Solid Edge part; units mm, degrees
sketch "Sketch1" plane through (0, 0, 0) normal (0, -1, 0) x (1, 0, 0)
  line L0 (38.9305, 51.9251) -> (68.9305, 51.9251)
  line L1 (68.9305, 51.9251) -> (68.9305, 21.9251)
  line L2 (68.9305, 21.9251) -> (38.9305, 21.9251)
  line L3 (38.9305, 21.9251) -> (38.9305, 51.9251)
  dimension "D1" = 38.9305
  dimension "D2" = 68.9305
extrude "Protrusion1" add sketch "Sketch1" against normal blind 15
sketch "Sketch2" plane through (63.9305, 0, 41.9251) normal (0, -1, 0) x (1, 0, 0)
  line L0 (-8, -5) -> (-8, -10)
  arc A0 (-8, -10) -> (-12, -10) centre (-10, -10) cw
  line L1 (-12, -10) -> (-12, -5)
  arc A1 (-12, -5) -> (-17, 0) centre (-17, -5) ccw
  line L2 (-17, 0) -> (-22, 0)
  arc A2 (-22, 0) -> (-22, 4) centre (-22, 2) cw
  line L3 (-22, 4) -> (-17, 4)
  arc A3 (-17, 4) -> (-14, 7) centre (-17, 7) ccw
  arc A4 (-14, 7) -> (-6, 7) centre (-10, 2.4867) cw
  arc A5 (-3, 4) -> (-6, 7) centre (-3, 7) cw
  line L4 (2, 4) -> (-3, 4)
  arc A6 (2, 0) -> (2, 4) centre (2, 2) ccw
  line L5 (-3, 0) -> (2, 0)
  arc A7 (-8, -5) -> (-3, 0) centre (-3, -5) cw
  dimension "D1" = 8
  dimension "D2" = 12
  dimension "D3" = 3
  dimension "D4" = 17
  dimension "D5" = 22
  dimension "D6" = 2
extrude "ExtrudedCutout_4" cut sketch "Sketch2" against normal blind 5
sketch "Sketch3" plane through (63.9305, 5, 35.4251) normal (0, -1, 0) x (1, 0, 0)
  circle A0 centre (-10, 8.5) radius 2.5
extrude "ExtrudedProtrusion_3" add sketch "Sketch3" along normal blind 5
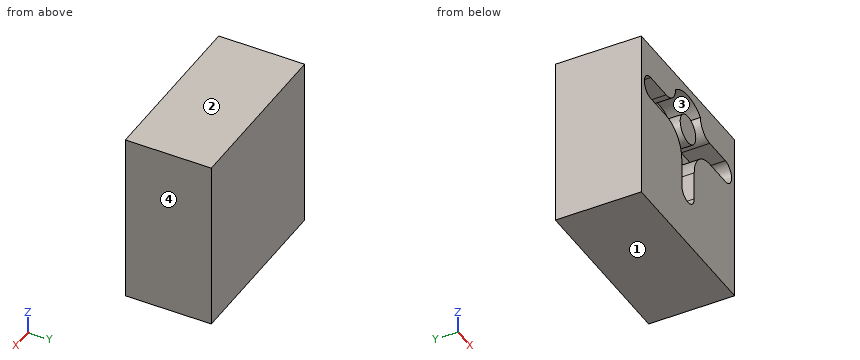
Source: CAD feature listing. Evaluate the final solid. Frame: model axes, mm. Face numbers are marked on the shaded views. Coordinates: 2 decimals unless noted, no trailing zeros. Loops run counter-clockwise (first coordinate to the right, second up) from the corner with the lowest first, then second, coordinate; pieces in that order, holes last. Notation, with made-up numbers: M 83,14.25 L 105,14.25 A20 ccw 105,35.25 Z; hole C -26,-32.5 d10. An arc over 180 degrees is marked long. Use a Markdown table: item, result. Add a question column.
Q1. Section query D-D, the plane x = 55. Return loops of the section in (y, z), and give its area (3 significant figures).
Q2. Draft query along Z for the marked faces 1, 2, 3 and 4. Return one class per face: pulls with the +Z half, pulls with the -Z half, needs draft (parallel to the pull), parting line crosses it, or undercut.
Q3. Material intervals for L1, parallel to Z at x = 41.75, y = 3.5; L2, parallel to X at y = 2.25, z = 42.5; L3, parallel to Y at x = 55.5, z = 37.75, sorted ascending.
Q4. Section query B-B, the plane z = 34.75. Return loops of the section in (x, y).
Q5. Section query C-C, the plane x = 45.75. Return loops of the section in (y, z).
Q6. Section query A-A, the plane y = 2.75. Return loops of the section in (x, z).
Result:
| question | item | result |
|---|---|---|
| 1 | outline | M 0,21.93 L 15,21.93 L 15,51.93 L 0,51.93 L 0,50.35 L 5,50.35 L 5,46.18 L 0,46.18 L 0,41.67 L 5,41.67 L 5,30.24 L 0,30.24 Z |
| 1 | area | 372 mm2 |
| 2 | face 1 | pulls with the -Z half |
| 2 | face 2 | pulls with the +Z half |
| 2 | face 3 | undercut |
| 2 | face 4 | needs draft |
| 3 | L1 | z = 21.93 to 41.93, 45.92 to 51.93 |
| 3 | L2 | x = 38.93 to 40.53, 51.88 to 55.98, 67.33 to 68.93 |
| 3 | L3 | y = 5 to 15 |
| 4 | outline | M 38.93,0 L 51.93,0 L 51.93,5 L 55.93,5 L 55.93,0 L 68.93,0 L 68.93,15 L 38.93,15 Z |
| 5 | outline | M 0,21.93 L 15,21.93 L 15,51.93 L 0,51.93 L 0,45.93 L 5,45.93 L 5,41.93 L 0,41.93 Z |
| 6 | outline | M 38.93,21.93 L 68.93,21.93 L 68.93,51.93 L 38.93,51.93 Z; C 53.93,43.93 d5; hole M 41.93,41.93 L 46.93,41.93 A5 cw 51.93,36.93 L 51.93,31.93 A2 ccw 55.93,31.93 L 55.93,36.93 A5 cw 60.93,41.93 L 65.93,41.93 A2 ccw 65.93,45.93 L 60.93,45.93 A3 cw 57.93,48.93 A6.03 ccw 49.93,48.93 A3 cw 46.93,45.93 L 41.93,45.93 A2 ccw Z |
